Input: part model. Units: mm. Frame: model coordinates. A direction names the side the tool comes from. Coordinates: 2 decimals unless noted, no trailing zeros. Loops run counter-clockwise (first coordinate to the right, second up) from the corner with the lowest first, then second, coordinate; pieces in that order, holes last.
Item 1: Pull-direction query (X, two-part tool) for faces 1 (the cylindrical face through (0.35, 14.57, -1.12)), 2 (the flat face through (0, 29.55, 1.4)), 3 (the cylindrical face through (-3.479, 18.617, -4.538)); classes: released by +X, released by -X, zero draft, split by the parting line, or undercut.
Item 2: Reachability of faces 4 (the flat face through (5, 24.187, 2)), 5 (the flat face through (-1, 0, 1)), 6 (the flat face through (5, 13.2, 0)) from +Z, -Z, +X, -X, +Y, -Y: full face, straight path, thin tool, end or side. Return the list, or none.
Item 3: Contact query for flat-ended pins moving along their axis: P1, Ø6, axis at x = -4, y = 6, coming from the +Z side; P2, Ø1.5, axis at y = 21.5, z = -2, coming from the +X side; P3, Ø2, axis at x = -2, y = 16.5, coming from the +Z side. Output: stop coordinate, or through.
Item 4: Section A-A on y = 9. Return loops of the section in (x, z) (3 decimals).
Item 5: Section B-B on y = 17.25. Return loops of the section in (x, z) (3 decimals), and give its area (3 significant figures).
Item 6: Ray query, line 1 along X through (y, z) = (14.5, 0) (3 decimals); line 2 along X through (y, z) = (12, 0) (3 decimals); line 3 along Y through (x, z) = (-3.5, -4). Return the intervals inside material, ascending.
```python
from build123d import *

# Parameters (mm, degrees)
SKETCH1_R           = 4.69
BOSS_EXTRUDE1_DEPTH = 13.2
SKETCH2_R           = 5.717952417
BOSS_EXTRUDE2_DEPTH = 16.35
SKETCH4_R           = 1.175
CUT_EXTRUDE1_DEPTH  = 31.636456479


with BuildPart() as part:
    # Sketch1 → Boss-Extrude1 (new body)
    with BuildSketch(Plane(origin=(0, 0, 0), x_dir=(1, 0, 0), z_dir=(0, 1, 0))):
        with Locations(Location((0, 0, 0), (0, 0, 270))):
            Circle(SKETCH1_R)
    extrude(amount=BOSS_EXTRUDE1_DEPTH)

    # Sketch2 → Boss-Extrude2 (add)
    with BuildSketch(Plane(origin=(0, 13.2, 0), x_dir=(1, 0, 0), z_dir=(0, 1, 0))):
        with Locations(Location((0, 0, 0), (0, 0, 270))):
            Circle(SKETCH2_R)
    extrude(amount=BOSS_EXTRUDE2_DEPTH)

    # Sketch3 → Cut-Revolve1 (revolve, cut)
    with BuildSketch(Plane.XY, mode=Mode.PRIVATE) as cut_revolve1_sk:
        with BuildLine():
            Line((3.297149576, 29.55), (5.717952417, 29.55))
            Line((5.717952417, 29.55), (5.717952417, 24.186874615))
            Line((5.717952417, 24.186874615), (5.202740875, 24.186874615))
            ThreePointArc((5.202740875, 24.186874615), (4.750212863, 27.046189194), (3.297149576, 29.55))
        make_face()
    revolve(cut_revolve1_sk.sketch.rotate(Axis((0, 29.55, 0), (0, -1, 0)), 90), axis=Axis((0, 29.55, 0), (0, -1, 0)), mode=Mode.SUBTRACT)

    # Sketch4 → Cut-Extrude1 (cut, through all)
    with BuildSketch(Plane.XZ):
        with Locations(Location((0, 0, 0), (0, 0, 270))):
            Circle(SKETCH4_R)
    extrude(amount=-CUT_EXTRUDE1_DEPTH, mode=Mode.SUBTRACT)


solid = part.part
```
Results found:
1. face 1: undercut
1. face 2: zero draft
1. face 3: split by the parting line
2. face 4: +Y
2. face 5: +Z, -Z, +X, -X, -Y
2. face 6: -Y
3. P1: stops at z = 4.58
3. P2: stops at x = 5.58
3. P3: stops at z = 5.63
4. outline: circle Ø9.38 at (0, 0); hole circle Ø2.35 at (0, 0)
5. outline: circle Ø11.436 at (0, 0); hole circle Ø2.35 at (0, 0)
5. area: 98.4 mm2
6. line 1: x = -5.718 to -1.175, 1.175 to 5.718
6. line 2: x = -4.69 to -1.175, 1.175 to 4.69
6. line 3: y = 13.2 to 24.19
